Can you work these out from the model? Positions are in its coordinate system, mm. Face numbers are marked on the shaded views. Give positions to 0.01 mm unless a question says otherwise; leave off trailing zeros. Write each loop counter-clockwise with the first axis right and the second up, starting at its lowest first coordinate (ties: lowest second). Pieces come first, ordered by that corner, then holes. Notation, with made-up numbers: (-28, 66) -> (31, 66) arc R18 ccw to (31, 82) -> close; hole circle Ø7 at (-27.75, -24). An arc over 180 degrees is marked (long way). One line per item, written item: value.
Autodesk Inventor part; units mm, degrees
ref_plane "YZ Plane" through (0, 0, 0) normal (1, 0, 0) x (0, 1, 0)
ref_plane "XZ Plane" through (0, 0, 0) normal (0, 1, 0) x (-1, 0, 0)
ref_plane "XY Plane" through (0, 0, 0) normal (0, 0, 1) x (1, 0, 0)
sketch "Sketch1" plane through (0, 0, 0) normal (0, 0, 1) x (1, 0, 0)
  line L0 (0, 0) -> (16.5, 0) construction
  line L1 (16.5, 0) -> (16.5, 7)
  line L2 (16.5, 7) -> (0, 7)
  line L3 (0, 7) -> (0, 9)
  line L4 (0, 9) -> (50, 9)
  line L5 (50, 9) -> (50, 0)
  line L6 (50, 0) -> (16.5, 0)
  line L7 (0, 7) -> (0, 0) construction
  dimension "d0" = 16.5
  dimension "d1" = 7
  dimension "d2" = 2
  dimension "d3" = 50
revolve "Revolution1" add sketch "Sketch1" angle 360 about axis through (0, 7, 0) along (0, 1, 0)
sketch "Sketch2" plane through (0, 0, 0) normal (0, -1, 0) x (1, 0, 0)
  line L0 (0, 20) -> (0, -20) construction
  line L1 (-4.2, 20) -> (-4.2, -20)
  line L2 (4.2, -20) -> (4.2, 20)
  arc A0 (4.2, 20) -> (-4.2, 20) centre (0, 20) ccw
  arc A1 (-4.2, -20) -> (4.2, -20) centre (0, -20) ccw
  line L3 (-20, 0) -> (20, 0) construction
  line L4 (-20, -4.2) -> (20, -4.2)
  line L5 (20, 4.2) -> (-20, 4.2)
  arc A2 (-20, 4.2) -> (-20, -4.2) centre (-20, 0) ccw
  arc A3 (20, -4.2) -> (20, 4.2) centre (20, 0) ccw
  point P0 (0, 0)
  point P1 (4.2, 4.2)
  point P2 (-4.2, 4.2)
  point P3 (-4.2, -4.2)
  point P4 (4.2, -4.2)
  dimension "d5" = 4.2
  dimension "d6" = 40
  dimension "d7" = 40
extrude "Extrusion1" cut sketch "Sketch2" against normal blind 1.5
sketch "Sketch3" plane through (0, 1.5, 0) normal (0, -1, 0) x (1, 0, 0)
  arc A0 (4.2, 20) -> (-4.2, 20) centre (0, 20) ccw
  circle A1 centre (0, 20) radius 1.7
  arc A2 (20, -4.2) -> (20, 4.2) centre (20, 0) ccw
  circle A3 centre (20, 0) radius 1.7
  arc A4 (-4.2, -20) -> (4.2, -20) centre (0, -20) ccw
  circle A5 centre (0, -20) radius 1.7
  arc A6 (-20, 4.2) -> (-20, -4.2) centre (-20, 0) ccw
  circle A7 centre (-20, 0) radius 1.7
  point P0 (0, 0)
  dimension "d10" = 3.4
extrude "Extrusion2" cut sketch "Sketch3" against normal through all
sketch "Sketch4" plane through (0, 9, 0) normal (0, 1, 0) x (1, 0, 0)
  circle A0 centre (0, -20) radius 1.7
  line L0 (-1.6454, -17.15) -> (1.6454, -17.15)
  line L1 (1.6454, -17.15) -> (3.2909, -20)
  line L2 (3.2909, -20) -> (1.6454, -22.85)
  line L3 (1.6454, -22.85) -> (-1.6454, -22.85)
  line L4 (-1.6454, -22.85) -> (-3.2909, -20)
  line L5 (-3.2909, -20) -> (-1.6454, -17.15)
  circle A1 centre (0, 20) radius 1.7
  line L6 (-1.6454, 17.15) -> (-3.2909, 20)
  line L7 (-3.2909, 20) -> (-1.6454, 22.85)
  line L8 (-1.6454, 22.85) -> (1.6454, 22.85)
  line L9 (1.6454, 22.85) -> (3.2909, 20)
  line L10 (3.2909, 20) -> (1.6454, 17.15)
  line L11 (1.6454, 17.15) -> (-1.6454, 17.15)
  circle A2 centre (20, 0) radius 1.7
  line L12 (21.6454, 2.85) -> (23.2909, 0)
  line L13 (23.2909, 0) -> (21.6454, -2.85)
  line L14 (21.6454, -2.85) -> (18.3546, -2.85)
  line L15 (18.3546, -2.85) -> (16.7091, 0)
  line L16 (16.7091, 0) -> (18.3546, 2.85)
  line L17 (18.3546, 2.85) -> (21.6454, 2.85)
  circle A3 centre (-20, 0) radius 1.7
  line L18 (-21.6454, 2.85) -> (-18.3546, 2.85)
  line L19 (-18.3546, 2.85) -> (-16.7091, 0)
  line L20 (-16.7091, 0) -> (-18.3546, -2.85)
  line L21 (-18.3546, -2.85) -> (-21.6454, -2.85)
  line L22 (-21.6454, -2.85) -> (-23.2909, 0)
  line L23 (-23.2909, 0) -> (-21.6454, 2.85)
  point P0 (0, 0)
  point P1 (0, -20)
  point P2 (0, 20)
  dimension "d13" = 5.7
extrude "Extrusion3" cut sketch "Sketch4" against normal blind 3.5 contours A0 | L0 L1 L2 L3 L4 L5 | A1 | L6 L7 L8 L9 L10 L11 | A2 | L12 L13 L14 L15 L16 L17 | A3 | L18 L19 L20 L21 L22 L23
chamfer "Chamfer1" distance 1 angle 45 2 edges at (-50, 0, 0) (-50, 9, 0)
chamfer "Chamfer2" distance 1 angle 45 4 edges at (-11.6673, 0, -11.6673) (-11.6673, 0, 11.6673) (11.6673, 0, 11.6673) (11.6673, 0, -11.6673)
properties part number "Platform"
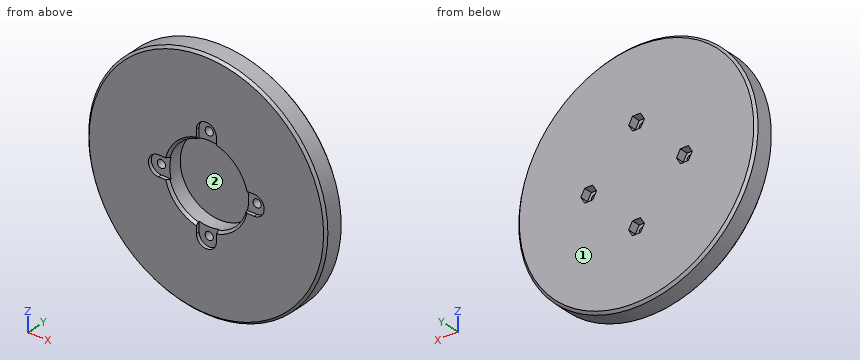
1) If we section it at B-B (y = 3.75): Write out the boundary of the cut face in (x, z).
Answer list:
outline: circle Ø100 at (0, 0); hole circle Ø3.4 at (-20, 0); hole circle Ø33 at (0, 0); hole circle Ø3.4 at (0, -20); hole circle Ø3.4 at (0, 20); hole circle Ø3.4 at (20, 0)
2) Will these pins go through, and if not, where does the flat tip stop? pin 1 (1 mm diameter, centred on x = -0.5, y = 8, fed in from +Z); pin 2 (4 mm diameter, centred on x = -2, z = -19, fed in from -Y); pin 3 (1.6 mm diameter, centred on x = -0.5, y = 7.5, fed in from -Z); pin 4 (4.5 mm diameter, centred on x = -0.5, z = -19, fed in from +Y).
Answer list:
pin 1: stops at z = 50
pin 2: stops at y = 1.5
pin 3: stops at z = -50
pin 4: stops at y = 9
3) I need wall thicknesses on L1, parallel to Z at x = 0, y = 4.65; L2, parallel to X at y = 3, z = -7.5; L3, parallel to Y at x = -3, z = -18. Which ranges of each line are inside material? Lowest first, please.
Answer list:
L1: z = -50 to -21.7, -18.3 to -16.5, 16.5 to 18.3, 21.7 to 50
L2: x = -49.43 to -14.7, 14.7 to 49.43
L3: y = 1.5 to 9
4) We'd pull the mould along Z, two halves only. Please class the marked faces 1 and 2: released by +Z, released by -Z, zero draft, split by the parting line, or undercut.
Answer list:
face 1: zero draft
face 2: undercut
5) If we section it at A-A (x = 0): State how many separate pieces and enclosed holes the cut face has, and give its area (3 significant figures).
Answer list:
separate pieces: 3
enclosed holes: 0
area: 577 mm^2
